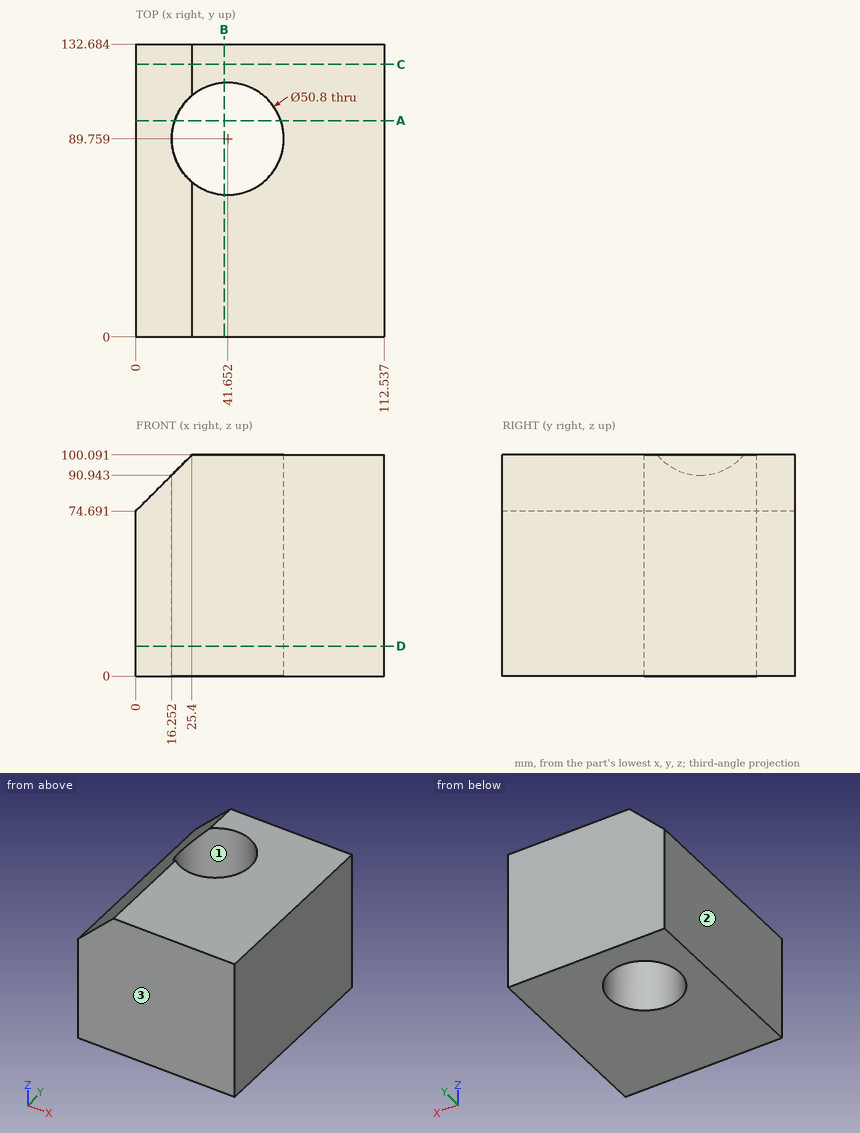
Study the drawing (mm; zero at the part's minimum x, y, z) and answer. Coordinates: 2 decimals unless noted, no trailing zeros. Loops run counter-clockwise (first coordinate to the right, second up) from the corner with the lowest first, then second, coordinate; pieces in that order, holes last. Notation, with made-up numbers: (12.25, -20.5) -> (41.25, -20.5) arc R13 cw to (41.25, -15.5) -> close; hole circle Ø3 at (88, 32). An arc over 180 degrees is marked (long way). Answer as CSV lines item,"result".
1) The part is cut by section B-B (x = 40). Give the vertices of the cut face in (y, z) (1 decimal), and give its area (3 significant figures).
A:
outline,"(0, 0) -> (64.4, 0) -> (64.4, 100.1) -> (0, 100.1) -> close; (115.1, 0) -> (132.7, 0) -> (132.7, 100.1) -> (115.1, 100.1) -> close"
area,"8,210 mm²"
2) The part is cut by section D-D (z = 13.5). Give the vertices of the cut face in (x, y) (1 decimal).
A:
outline,"(0, 0) -> (112.5, 0) -> (112.5, 132.7) -> (0, 132.7) -> close; hole circle Ø50.8 at (41.7, 89.8)"
3) The part is cut by section A-A (y = 98). Give the vertices of the cut face in (x, z), and give its area (3 significant figures).
A:
outline,"(0, 0) -> (17.63, 0) -> (17.63, 92.32) -> (0, 74.69) -> close; (65.68, 0) -> (112.54, 0) -> (112.54, 100.09) -> (65.68, 100.09) -> close"
area,"6,160 mm²"
4) The part is cut by section C-C (y = 123.5). Give the vertices of the cut face in (x, z).
A:
outline,"(0, 0) -> (112.54, 0) -> (112.54, 100.09) -> (25.4, 100.09) -> (0, 74.69) -> close"
5) For a pull along Y with two mould halves and no side action, classify the marked faces 1, 2 and 3 as released by +Y, released by -Y, zero draft, split by the parting line, or undercut.
A:
face 1,"undercut"
face 2,"zero draft"
face 3,"released by -Y"
6) Straight lines are drawn through the part: probe 1 along Y at (x, z) = (24, 14.5) (1 decimal); probe 2 along X at (y, z) = (92, 16); probe 3 along Y at (x, z) = (30.5, 11.5) (1 decimal). For each, find the intervals that lie inside material, in ascending order.
A:
probe 1,"y = 0 to 71.5, 108 to 132.7"
probe 2,"x = 0 to 16.35, 66.95 to 112.54"
probe 3,"y = 0 to 66.9, 112.6 to 132.7"
